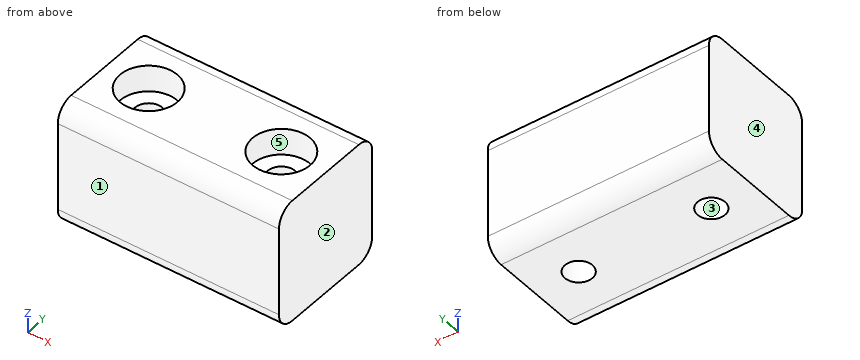
Autodesk Inventor part; units mm, degrees
ref_plane "YZ Plane" through (0, 0, 0) normal (1, 0, 0) x (0, 1, 0)
ref_plane "XZ Plane" through (0, 0, 0) normal (0, 1, 0) x (-1, 0, 0)
ref_plane "XY Plane" through (0, 0, 0) normal (0, 0, 1) x (1, 0, 0)
sketch "Sketch1" plane through (0, 0, 0) normal (0, 0, 1) x (1, 0, 0)
  line L0 (-12.5, 7) -> (12.5, 7)
  line L1 (12.5, 7) -> (12.5, -7)
  line L2 (12.5, -7) -> (-12.5, -7)
  line L3 (-12.5, -7) -> (-12.5, 7)
  point P0 (0, 0)
  point P1 (12.5, 0)
  point P2 (0, 7)
  dimension "d0" = 25
  dimension "d2" = 14
extrude "Extrusion1" add sketch "Sketch1" along normal blind 14
sketch "Sketch2" plane through (0, 0, 14) normal (0, 0, 1) x (1, 0, 0)
  line L0 (-7.5, 0) -> (7.5, 0)
  point P0 (0, 0)
  point P1 (0, 0)
  dimension "d5" = 15
hole "Hole1" at (-7.5, 0, 14) at (7.5, 0, 14) direction (0, 0, -1) diameter 3.1 end through all counterbore diameter 6.5 counterbore depth 3
fillet "Fillet1" radius 2 2 edges at (0, 7, 0) (0, -7, 0)
fillet "Fillet2" radius 2 2 edges at (0, 7, 14) (0, -7, 14)
properties part number "string tensioner"
Could you check a few things on this model? Use its own coordinates, in mm. Face numbers are marked on the shaded views. A direction names the side the tool comes from. Coordinates: 2 decimals unless noted, no trailing zeros. Loops run counter-clockwise (first coordinate to the right, second up) from the corner with the lowest first, then second, coordinate; pieces in that order, holes last. Notation, with made-up numbers: (4, -7) -> (28, -7) arc R5 ccw to (28, 1) -> close; hole circle Ø2 at (8, 58.25). An arc over 180 degrees is marked (long way). Answer in a Markdown table with one row per item.
(1) If I drill on probe 1 along X at (y, z) = (0, 12.9); probe 2 along X at (y, z) = (0, 6.75); probe 3 along Y at (x, z) = (-7.5, 11.85), over which ranges is the centre line in solid material (lowest first)?
Results found:
| item | result |
|---|---|
| probe 1 | x = -12.5 to -10.75, -4.25 to 4.25, 10.75 to 12.5 |
| probe 2 | x = -12.5 to -9.05, -5.95 to 5.95, 9.05 to 12.5 |
| probe 3 | y = -7 to -3.25, 3.25 to 7 |
(2) Imagine slicing it at A-A (x = 7.5). List the corners of the cut face in (y, z) for me, plus the area to 3 significant figures.
Results found:
| item | result |
|---|---|
| outline | (-7, 2) arc R2 ccw to (-5, 0) -> (-1.55, 0) -> (-1.55, 11) -> (-3.25, 11) -> (-3.25, 14) -> (-5, 14) arc R2 ccw to (-7, 12) -> close; (1.55, 0) -> (5, 0) arc R2 ccw to (7, 2) -> (7, 12) arc R2 ccw to (5, 14) -> (3.25, 14) -> (3.25, 11) -> (1.55, 11) -> close |
| area | 139 mm^2 |
(3) Imagine slicing it at C-C (x = -0.75). List the corners of the cut face in (y, z) for me.
Results found:
| item | result |
|---|---|
| outline | (-7, 2) arc R2 ccw to (-5, 0) -> (5, 0) arc R2 ccw to (7, 2) -> (7, 12) arc R2 ccw to (5, 14) -> (-5, 14) arc R2 ccw to (-7, 12) -> close |
(4) Imagine slicing it at B-B (z = 4.5). List the corners of the cut face in (x, y) for me.
Results found:
| item | result |
|---|---|
| outline | (-12.5, -7) -> (12.5, -7) -> (12.5, 7) -> (-12.5, 7) -> close; hole circle Ø3.1 at (-7.5, 0); hole circle Ø3.1 at (7.5, 0) |
(5) Thinking about a two-plate mould opening in X: for the marked faces 1, 2 and 3, which applies, released by +X, released by -X, zero draft, split by the parting line, or undercut?
Results found:
| item | result |
|---|---|
| face 1 | zero draft |
| face 2 | released by +X |
| face 3 | undercut |
(6) Imagine slicing it at D-D (y = -1.25). List the corners of the cut face in (x, z) for me, plus the area to 3 significant figures.
Results found:
| item | result |
|---|---|
| outline | (-12.5, 0) -> (-8.42, 0) -> (-8.42, 11) -> (-10.5, 11) -> (-10.5, 14) -> (-12.5, 14) -> close; (-6.58, 0) -> (6.58, 0) -> (6.58, 11) -> (4.5, 11) -> (4.5, 14) -> (-4.5, 14) -> (-4.5, 11) -> (-6.58, 11) -> close; (8.42, 0) -> (12.5, 0) -> (12.5, 14) -> (10.5, 14) -> (10.5, 11) -> (8.42, 11) -> close |
| area | 274 mm^2 |
(7) Will this pin go through, and if not, where does the flat tip stop? pin 1 Ø4 at (x, y) = (-7.5, 0) entering from +Z.
Results found:
| item | result |
|---|---|
| pin 1 | stops at z = 11 |
(8) For the marked faces 4 and 5, which set-ups out of +Z, -Z, +X, -X, +Y, -Y let a thin tool reach every point of the face, with its end or its side?
Results found:
| item | result |
|---|---|
| face 4 | +Z, -Z, -X, +Y, -Y |
| face 5 | +Z |
